The model under review builds one solid part; all positions refer to its coordinate system, in mm. A direction names the side the tool comes from. Round coordinates to 2 decimals unless told otherwise and drop trailing zeros. Write each loop counter-clockwise with the first axis right and the second up, starting at its lowest first coordinate (ties: lowest second). Pieces come first, ordered by that corner, then holes.
Item 1: Add section C-C (x = -10). Give the boundary of the cut face in (y, z).
Item 2: Machinability: for faces 1 (the face through (-12.15, -9, -25)), 2 (the face through (-1, -35, -25)), which of the approach directions +Z, -Z, +X, -X, +Y, -Y give a long, thin tool a straight path to every point of the face, cutting with its end or side? Answer none if there is none.
Item 3: Add section D-D (z = 17). Give the boundary of the cut face in (x, y), plus the area to 3 significant figures.
Item 4: Add section A-A (y = -26.85). Give the boundary of the cut face in (x, z), plus the area to 3 significant figures.
Item 5: To check wall thickness, follow L1, parallel to Y at x = -10, z = -24.8; L2, parallel to Z at x = -16, y = -1.2; L3, parallel to Z at x = 16, y = -1. State the ranges of each line that lie inside material, in increasing order.
Item 6: Clearance check with flat-ended pins moving along their axes: pin 1 Ø4 at (x, y) = (-10, -26.85) entering from +Z; pin 2 Ø2 at (y, z) = (-19, -24) entering from +X; pin 3 Ø1 at (x, y) = (8.5, -1) entering from -Z; pin 4 Ø4.5 at (x, z) = (-16, -16) entering from -Y. State where each tip first meets the part, or that it passes through.
Item 7: Draft analysis for pull direction Y (two halves, no side actions). For faces 3 (the face through (-6, 0, -18.2)), 4 (the face through (-9.9, -16.7, -25)), 5 (the face through (0, -16, -25)), state which applies: +Y half, -Y half, draft (parallel to the pull), parting line (faces both ways), or undercut.
Item 8: Add section B-B (z = 0). Give the boundary of the cut face in (x, y).
```python
from build123d import *

# Parameters (mm, degrees)
F0_W     = 40
F0_H     = 40
F0_R     = 2
F0_R_2   = 19
F1_DEPTH = 2
F2_W     = 20
F2_H     = 2
F3_DEPTH = 6
F4_W     = 20
F4_H     = 37
F5_DEPTH = 2
F6_R     = 5
F7_R     = 2.15
F8_DEPTH = 3
F9_R     = 2


with BuildPart() as f1:
    # F0 (on Front) → F1 (new body)
    with BuildSketch(Plane.XZ):
        Rectangle(F0_W, F0_H)
        with Locations((-16, -16)):
            Circle(F0_R, mode=Mode.SUBTRACT)
        with Locations((16, -16)):
            Circle(F0_R, mode=Mode.SUBTRACT)
        with Locations((-16, 16)):
            Circle(F0_R, mode=Mode.SUBTRACT)
        Circle(F0_R_2, mode=Mode.SUBTRACT)
        with Locations((16, 16)):
            Circle(F0_R, mode=Mode.SUBTRACT)
    extrude(amount=F1_DEPTH)

    # F2 (on face) → F3 (join)
    with BuildSketch(Plane(origin=(0, 0, -20), x_dir=(1, 0, 0), z_dir=(0, 0, -1))):
        with Locations((-10, 1)):
            Rectangle(F2_W, F2_H)
    extrude(amount=F3_DEPTH)

    # F4 (on face) → F5 (join)
    with BuildSketch(Plane(origin=(0, 0, -26), x_dir=(1, 0, 0), z_dir=(0, 0, -1))):
        with Locations((-10, 18.5)):
            Rectangle(F4_W, F4_H)
    extrude(amount=-F5_DEPTH)

    # F6
    f6_edges = [f1.edges().sort_by_distance(p)[0] for p in [
        (20, -1, -20),
        (20, -1, 20),
        (-20, -1, 20),
        (-20, -37, -25),
        (0, -37, -25),
    ]]
    fillet(f6_edges, radius=F6_R)

    # F7 (on face) → F8 (cut)
    with BuildSketch(Plane(origin=(0, 0, -26), x_dir=(1, 0, 0), z_dir=(0, 0, -1))):
        with Locations((-10, 26.85)):
            Circle(F7_R)
        with BuildLine():
            Line((-12.15, 10.438207), (-12.15, 7.55))
            ThreePointArc((-12.15, 7.55), (-10, 5.4), (-7.85, 7.55))
            Line((-7.85, 7.55), (-7.85, 10.438207))
            ThreePointArc((-7.85, 10.438207), (-10, 16.7), (-12.15, 10.438207))
        make_face()
    extrude(amount=-F8_DEPTH, mode=Mode.SUBTRACT)

    # F9
    f9_edges = [f1.edges().sort_by_distance(p)[0] for p in [
        (0, -1, -20),
        (-10, 0, -26),
    ]]
    fillet(f9_edges, radius=F9_R)


solid = f1.part
```
Numbers:
1. outline: (-37, -26) - (-29, -26) - (-29, -24) - (-37, -24) - close; (-24.7, -26) - (-16.7, -26) - (-16.7, -24) - (-24.7, -24) - close; (-5.4, -26) - (-2, -26) arc R2 ccw to (0, -24) - (0, -16.16) - (-2, -16.16) - (-2, -24) - (-5.4, -24) - close; (-2, 16.16) - (0, 16.16) - (0, 20) - (-2, 20) - close
2. face 1: +Z, -Z
2. face 2: +Z, -Z, +X, -Y
3. outline: (-19.58, -2) - (-17.73, -2) - (-17.73, 0) - (-19.58, 0) - close; (-14.27, -2) - (-8.49, -2) - (-8.49, 0) - (-14.27, 0) - close; (8.49, -2) - (14.27, -2) - (14.27, 0) - (8.49, 0) - close; (17.73, -2) - (19.58, -2) - (19.58, 0) - (17.73, 0) - close
3. area: 30.5 mm2
4. outline: (-20, -26) - (-12.15, -26) - (-12.15, -24) - (-20, -24) - close; (-7.85, -26) - (0, -26) - (0, -24) - (-7.85, -24) - close
4. area: 31.4 mm2
5. L1: y = -37 to -29, -24.7 to -16.7, -5.4 to -0.17
5. L2: z = -25.83 to -18, -14 to -10.25, 10.25 to 14, 18 to 19.9
5. L3: z = -19.9 to -18, -14 to -10.25, 10.25 to 14, 18 to 19.9
6. pin 1: passes through
6. pin 2: stops at x = 0
6. pin 3: stops at z = -20
6. pin 4: stops at y = -2
7. face 3: +Y half
7. face 4: undercut
7. face 5: draft
8. outline: (-20, -2) - (-19, -2) - (-19, 0) - (-20, 0) - close; (19, -2) - (20, -2) - (20, 0) - (19, 0) - close
